The model under review builds one solid part; all positions refer to its coordinate system, in mm. A direction names the side the tool comes from. Give positions to 0.01 mm unless a question says otherwise; leave off trailing zeros. Order: outer loops, then holes, each group sorted by start corner. A loop starts at its lowest first (then second) coordinate and runs counter-clockwise, first axis right, second up. Notation, with made-up numbers: (-31, -3.5) -> (-18, -3.5) arc R23 ccw to (-18, 4.5) -> close; hole circle Ø9 at (43.5, 18.5). An arc over 180 degrees is marked (long way). Use one line per item in the form item = value.
```python
from build123d import *

# Parameters (mm, degrees)
BASPROSKE_W         = 10
BASPROSKE_H         = 6.86
TOOTHCUT_DEPTH      = 14.932666651
TEETHCUTS_COUNT     = 12
TEETHCUTS_ANGLE     = 330
BORSKE_R            = 1
BORE_DEPTH          = 50.0000508
SKETCH1_R           = 12.5
BOSS_EXTRUDE1_DEPTH = 6
SKETCH2_R           = 1.65
CUT_EXTRUDE1_DEPTH  = 21.310096012
SKETCH3_R           = 3
CUT_EXTRUDE2_DEPTH  = 4
CIRPATTERN1_COUNT   = 4
CHAMFER1_SIZE       = 4
SKETCH4_R           = 2.25
CUT_EXTRUDE3_DEPTH  = 6


with BuildPart() as part:
    # BasProSke → Base-Revolve (revolve)
    with BuildSketch(Plane(origin=(0, 0, 0), x_dir=(1, 0, 0), z_dir=(0, 1, 0)), mode=Mode.PRIVATE) as base_revolve_sk:
        with Locations((5, 3.43)):
            Rectangle(BASPROSKE_W, BASPROSKE_H)
    revolve(base_revolve_sk.sketch.rotate(Axis((-10, 0, 0), (1, 0, 0)), 180), axis=Axis((-10, 0, 0), (1, 0, 0)))

    # TooCutSke → ToothCut (cut, through all)
    with BuildSketch(Plane(origin=(0, 0, 0), x_dir=(0, 0, -1), z_dir=(1, 0, 0))):
        with BuildLine():
            ThreePointArc((0.552016647, 4.621146354), (0, 4.654), (-0.552016647, 4.621146354))
            ThreePointArc((-0.552016647, 4.621146354), (-0.822258441, 5.798784691), (-1.641510828, 6.686865885))
            ThreePointArc((-1.641510828, 6.686865885), (0, 6.8854), (1.641510828, 6.686865885))
            ThreePointArc((1.641510828, 6.686865885), (0.822258441, 5.798784691), (0.552016647, 4.621146354))
        make_face()
    toothcut = extrude(amount=TOOTHCUT_DEPTH, mode=Mode.SUBTRACT)

    # TeethCuts: ToothCut ×12 about axis
    teethcuts_axis = Axis((-10, 0, 0), (1, 0, 0))
    for i in range(1, TEETHCUTS_COUNT):
        add(toothcut.rotate(teethcuts_axis, i * TEETHCUTS_ANGLE / (TEETHCUTS_COUNT - 1)), mode=Mode.SUBTRACT)

    # BorSke → Bore (cut, symmetric)
    with BuildSketch(Plane(origin=(0, 0, 0), x_dir=(0, 0, -1), z_dir=(1, 0, 0))):
        with Locations(Location((0, 0, 0), (0, 0, 180))):
            Circle(BORSKE_R)
    extrude(amount=BORE_DEPTH, both=True, mode=Mode.SUBTRACT)

    # Sketch1 → Boss-Extrude1 (add)
    with BuildSketch(Plane(origin=(10, 0, 0), x_dir=(0, 0, -1), z_dir=(1, 0, 0))):
        Circle(SKETCH1_R)
    extrude(amount=BOSS_EXTRUDE1_DEPTH)

    # Sketch2 → Cut-Extrude1 (cut, through all)
    with BuildSketch(Plane.ZY.offset(-10)):
        with Locations((0, 9)):
            Circle(SKETCH2_R)
    cut_extrude1 = extrude(amount=-CUT_EXTRUDE1_DEPTH, mode=Mode.SUBTRACT)

    # Sketch3 → Cut-Extrude2 (cut)
    with BuildSketch(Plane.ZY.offset(-10)):
        with Locations((0, 9)):
            Circle(SKETCH3_R)
    cut_extrude2 = extrude(amount=-CUT_EXTRUDE2_DEPTH, mode=Mode.SUBTRACT)

    # CirPattern1: Cut-Extrude1, Cut-Extrude2 ×4 about axis
    cirpattern1_axis = Axis((0, 0, 0), (1, 0, 0))
    add([cut_extrude1.rotate(cirpattern1_axis, i * 360 / CIRPATTERN1_COUNT) for i in range(1, CIRPATTERN1_COUNT)], mode=Mode.SUBTRACT)
    add([cut_extrude2.rotate(cirpattern1_axis, i * 360 / CIRPATTERN1_COUNT) for i in range(1, CIRPATTERN1_COUNT)], mode=Mode.SUBTRACT)

    # Chamfer1
    # the kernel refuses this chamfer: 4 mm, written as the material it takes off along each edge
    with BuildSketch(Plane(origin=(10, 0, 0), x_dir=(0, 0, -1), z_dir=(0, -1, 0))) as chamfer1_piece_1:
        Polygon((12.5, CHAMFER1_SIZE), (12.5 - CHAMFER1_SIZE, 0), (12.5, 0), align=None)
    revolve(axis=Axis((10, 0, 0), (1, 0, 0)), mode=Mode.SUBTRACT)

    # Sketch4 → Cut-Extrude3 (cut)
    with BuildSketch(Plane(origin=(16, 0, 0), x_dir=(0, 0, -1), z_dir=(1, 0, 0))):
        Circle(SKETCH4_R)
    extrude(amount=-CUT_EXTRUDE3_DEPTH, mode=Mode.SUBTRACT)


solid = part.part
```
1. Add section A-A on z = 0. Count the separate pieces of the cut face and the enclosed holes in it, then the cut area to 3 significant figures.
Values:
separate_pieces = 4
enclosed_holes = 0
area = 131 mm^2
2. Tool access review of faces 1 (the face through (12.42, 0.65, 6.07)), 2 (the face through (10, -1, 1)): name each direction out of +Z, -Z, +X, -X, +Y, -Y from which nothing blocks a thin tool from reaching the whole face with its end or side.
Values:
face_1 = none
face_2 = +X
3. Add section B-B on x = 14.75. Give the boundary of the cut face in (y, z).
Values:
outline = circle Ø25 at (0, 0); hole circle Ø3.3 at (-9, 0); hole circle Ø4.5 at (0, 0); hole circle Ø3.3 at (0, -9); hole circle Ø3.3 at (0, 9); hole circle Ø3.3 at (9, 0)
4. For L1, parallel to Y at x = 13.1, z = 0; L2, parallel to Z at x = 5.5, y = 4.75; L3, parallel to X at y = 2.5, z = 7.5, list the stretches that pass through material, from the lowest coordinate up.
Values:
L1 = -6 to -2.25, 2.25 to 6
L2 = -4.95 to -3.87, -2.06 to -0.55, 0.55 to 2.06, 3.87 to 4.95
L3 = 14 to 16
5. For pin 1 Ø5 at (x, y) = (2.5, 7) entering from +Z; pin 2 Ø1 at (x, y) = (6.5, -6.5) entering from -Z; pin 3 Ø3 at (y, z) = (-5.5, 5.5) entering from -X; pin 4 Ø3 at (y, z) = (-0.5, 9) entering from -X, all flat-tipped, find the tip position at first contact; note any pin that passes through.
Values:
pin_1 = 4.97
pin_2 = -2.14
pin_3 = 0
pin_4 = 14
6. The part is to be moulded in two halves that separate along Z. For faces 3 (the face through (10.194, -3.33, -8.031)), 4 (the face through (4.93, -5.798, 0.822)), say which applies: +Z half, -Z half, draft (parallel to the pull), parting line (faces both ways), or undercut.
Values:
face_3 = parting line
face_4 = undercut
